Could you check a few things on this model? Use its own coordinates, in mm. Give positions to 0.01 mm unless a question says otherwise; leave off trailing zeros. Loops run counter-clockwise (first coordinate to the right, second up) from the corner with the lowest first, then second, coordinate; pieces in that order, holes last. Notation, with made-up numbers: M -33.5,-14 L 24.5,-14 A29 ccw 24.5,24 Z; hole C 71,-11.5 d9. An arc over 180 degrees is marked long. Return JSON: item names as keys, results as strings. Group by question number.
1. If we mould it in two halves opening along X, with no side actions, what happens to faces 1 (the cylindrical face through (15.286, 18.956, -6.494)), 2 (the flat face through (7, 20, 7)), 3 (the cylindrical face through (3.55, -6.31, 20.03))? For each: +X half, -X half, draft (parallel to the pull), parting line (faces both ways), or undercut.
2. If we section it at A-A (y = 0): Write out the boundary of the cut face in (x, z), plus the area to 3 significant figures.
3. If we section it at C-C (y = 24.5): Write out the boundary of the cut face in (x, z), plus the area to 3 significant figures.
4. Please list where these lines run through material, in increasing order: line 1 (X direction, y = 17.5, z = 0); line 2 (X direction, y = 23, z = 0); line 3 (Z direction, x = 15, y = 15).
5. If we section it at B-B (x = 39): Write out the boundary of the cut face in (y, z).
6. For pin 1 (3 mm diameter, centred on y = -9, z = 16, fed in from +X); pin 2 (6 mm diameter, centred on x = 24, y = 1.5, fed in from +Z); pin 3 (12 mm diameter, centred on y = 23, z = 5.5, fed in from +X), each with a flat end and sliding along its axis, tell me the tip position at first contact or that it passes through.
7. If we section it at D-D (x = 15): Write out the boundary of the cut face in (y, z), plus the area to 3 significant figures.
```python
from build123d import *

# Parameters (mm, degrees)
BOSS_EXTRU_1_REACH           = 74.101
ESQUISSE2_R                  = 8
ENL_V_MAT_EXTRU_1_REACH      = 74.101
ENL_V_MAT_EXTRU_1_END_RADIUS = 10
ESQUISSE3_R                  = 6.5


with BuildPart() as part:
    # Esquisse1 → Révolution1 (revolve)
    with BuildSketch(Plane.XY, mode=Mode.PRIVATE) as r_volution1_sk:
        Polygon((44, 10), (0, 10), (0, 21), (7, 21), (7, 22.5), (10, 22.5), (10, 15), (28, 15), (44, 11), align=None)
    revolve(r_volution1_sk.sketch.rotate(Axis((0, 0, 0), (1, 0, 0)), 90), axis=Axis((0, 0, 0), (1, 0, 0)))

    # Esquisse2 → Boss.-Extru.1 (add, up to next)
    with BuildSketch(Plane(origin=(0, 30, 0), x_dir=(1, 0, 0), z_dir=(0, 1, 0)), mode=Mode.PRIVATE) as boss_extru_1_sk1:
        with Locations(Location((15, 0, 0), (0, 0, 270))):
            Circle(ESQUISSE2_R)
    boss_extru_1_tool1 = extrude(boss_extru_1_sk1.sketch, amount=-BOSS_EXTRU_1_REACH, mode=Mode.PRIVATE) - part.part
    add(boss_extru_1_tool1.solids().sort_by_distance((15, 30, 0))[0])

    # Enlèv. mat.-Extru.1: up to this cylinder (the profile starts outside it)
    enl_v_mat_extru_1_end = Plane(origin=(15, 0, 0), z_dir=(-1, 0, 0)) * Cylinder(ENL_V_MAT_EXTRU_1_END_RADIUS, 169.202, mode=Mode.PRIVATE)
    # Esquisse3 → Enlèv. mat.-Extru.1 (cut, up to the surface)
    with BuildSketch(Plane(origin=(0, 30, 0), x_dir=(1, 0, 0), z_dir=(0, 1, 0)), mode=Mode.PRIVATE) as enl_v_mat_extru_1_sk1:
        with Locations(Location((15, 0, 0), (0, 0, 270))):
            Circle(ESQUISSE3_R)
    enl_v_mat_extru_1_tool1 = extrude(enl_v_mat_extru_1_sk1.sketch, amount=-ENL_V_MAT_EXTRU_1_REACH, mode=Mode.PRIVATE) - enl_v_mat_extru_1_end
    add(enl_v_mat_extru_1_tool1.solids().sort_by_distance((15, 30, 0))[0], mode=Mode.SUBTRACT)


solid = part.part
```
Answer:
{
 "1": {"face 1": "undercut", "face 2": "-X half", "face 3": "draft"},
 "2": {"outline": "M 0,-21 L 7,-21 L 7,-22.5 L 10,-22.5 L 10,-15 L 28,-15 L 44,-11 L 44,-10 L 0,-10 Z; M 0,10 L 44,10 L 44,11 L 28,15 L 10,15 L 10,22.5 L 7,22.5 L 7,21 L 0,21 Z", "area": "505 mm²"},
 "3": {"outline": "C 15,0 d16; hole C 15,0 d13", "area": "68.3 mm²"},
 "4": {"line 1": "x = 0 to 8.5, 21.5 to 23", "line 2": "x = 7 to 8.5, 21.5 to 23", "line 3": "z = -8 to -6.5, 6.5 to 8"},
 "5": {"outline": "C 0,0 d24.5; hole C 0,0 d20"},
 "6": {"pin 1": "stops at x = 10", "pin 2": "stops at z = 15", "pin 3": "stops at x = 23"},
 "7": {"outline": "M 7.6,-6.5 A10 cw long 7.6,6.5 L 30,6.5 L 30,8 L 12.69,8 A15 ccw long 12.69,-8 L 30,-8 L 30,-6.5 Z", "area": "375 mm²"}
}
